Here's the drawing with two shaded views (mm, measured from the low corner). I have some questions. A direction names the side the tool comes from. Round coordinates to 2 decimals unless told otherwise and drop trailing zeros. Order: outer loops, then holes, each group sorted by start corner. A loop starts at its lowest first (then second) coordinate and runs counter-clockwise, first axis right, second up. Notation, with made-up numbers: M 25.5,25 L 83.5,25 A13 ccw 83.5,41 Z; hole C 37,78 d8. An arc over 180 degrees is marked long. One line per question, with ' | ' between items.
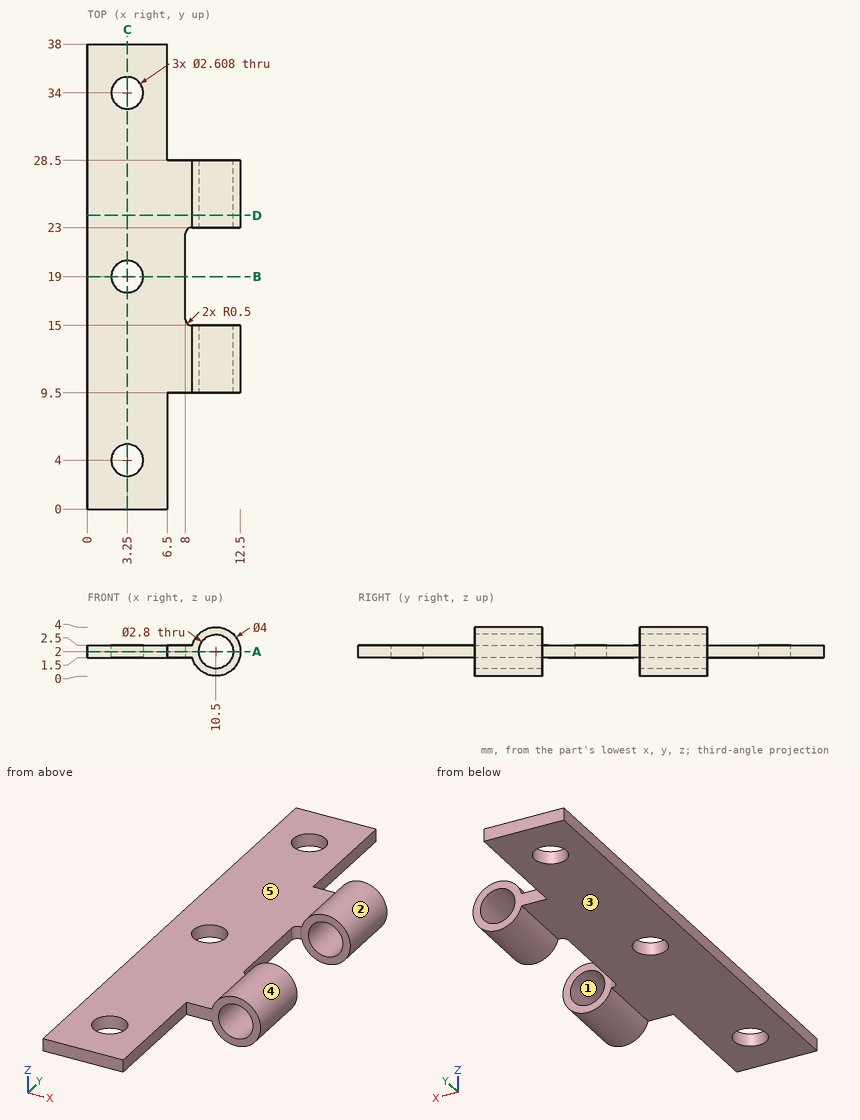
(1) If we section it at D-D on y = 24: Please give me the cut outline in (x, z).
Final values:
outline: M 0,1.5 L 8.56,1.5 A2 ccw long 8.56,2.5 L 0,2.5 Z; hole C 10.5,2 d2.8
(2) Please list where these lines run through material, in increasing order: probe 1 along Y at (x, z) = (3.25, 1.95); probe 2 along Y at (x, z) = (10.5, 3.85); probe 3 along Z at (x, y) = (10.5, 25.6). Write a range as [from, to].
Final values:
probe 1: [0, 2.7], [5.3, 17.7], [20.3, 32.7], [35.3, 38] | probe 2: [9.5, 15], [23, 28.5] | probe 3: [0, 0.6], [3.4, 4]
(3) If we section it at B-B on y = 19: Please give me the cut outline in (x, z).
Final values:
outline: M 0,1.5 L 1.95,1.5 L 1.95,2.5 L 0,2.5 Z; M 4.55,1.5 L 8,1.5 L 8,2.5 L 4.55,2.5 Z
(4) If we section it at A-A on z = 2: Please give me the cut outline in (x, y).
Final values:
outline: M 0,0 L 6.5,0 L 6.5,9.5 L 9.1,9.5 L 9.1,15 L 8.5,15 A0.5 cw 8,15.5 L 8,22.5 A0.5 cw 8.5,23 L 9.1,23 L 9.1,28.5 L 6.5,28.5 L 6.5,38 L 0,38 Z; M 11.9,9.5 L 12.5,9.5 L 12.5,15 L 11.9,15 Z; M 11.9,23 L 12.5,23 L 12.5,28.5 L 11.9,28.5 Z; hole C 3.25,4 d2.61; hole C 3.25,19 d2.61; hole C 3.25,34 d2.61
(5) Will these pins go through, and if not, where does the flat tip stop? pin 1 Ø1.5 at (x, y) = (4, 22.5) entering from +Z; pin 2 Ø4 at (x, y) = (3.25, 34) entering from -Z; pin 3 Ø0.5 at (y, z) = (6, 2) entering from +X.
Final values:
pin 1: z = 2.5 | pin 2: z = 1.5 | pin 3: x = 6.5
(6) Thinking about a two-plate mould opening in Z: for the marked faces 1, 2 and 3, which applies, released by +Z, released by -Z, zero draft, split by the parting line, or undercut?
Final values:
face 1: undercut | face 2: split by the parting line | face 3: released by -Z
(7) If we section it at C-C on x = 3.25: Please give me the cut outline in (y, z).
Final values:
outline: M 0,1.5 L 2.7,1.5 L 2.7,2.5 L 0,2.5 Z; M 5.3,1.5 L 17.7,1.5 L 17.7,2.5 L 5.3,2.5 Z; M 20.3,1.5 L 32.7,1.5 L 32.7,2.5 L 20.3,2.5 Z; M 35.3,1.5 L 38,1.5 L 38,2.5 L 35.3,2.5 Z
(8) On a 3-axis mill with a long thin cutter (end or side, diameter ignored), from which of +Z, -Z, +X, -X, +Y, -Y can I reach the whole of each face in a straight line? I mean the marked faces 4 and 5. Say none if no direction works.
Final values:
face 4: +Y, -Y | face 5: +Z, -X, +Y, -Y
